Here's how the part is built. I have some questions about the finished solid (model axes, mm). Round coordinates to 2 decimals unless told otherwise and drop trailing zeros. Order: outer loops, then holes, each group sorted by start corner. A loop starts at its lowest first (then second) coordinate and runs counter-clockwise, first axis right, second up. Notation, with made-up numbers: M 48.5,4 L 78.5,4 A16 cw 78.5,8 Z; hole C -13.5,-5.75 d7. An arc over 180 degrees is marked long. Write item = value, one per line. Start each with the question number.
Item 1: I want a section at A-A, the plane z = 0. List the corners of the cut face in (x, y) for me (3 decimals), plus the area to 3 significant figures.
Item 2: Please list where these lines run through material, in increasing order: L1, parallel to Z at x = -0.25, y = -2.8; L2, parallel to X at y = -4.5, z = -0.75; L3, parallel to X at y = -4.1, z = -1.25.
Item 3: I'm going to push flat-ended pins straight in: P1, Ø3, axis at y = -1, z = -1, coming from the -X side; P2, Ø1.5, axis at x = 1.5, y = -3.5, coming from the -Z side; P3, Ø1, axis at x = 3, z = 5.5, coming from the +Y side. Where does each tip first touch, or does it pass through?
Item 4: I want a section at B-B, the plane x = 0. List the corners of the cut face in (y, z) for me (3 decimals), plus the area to 3 significant figures.
Item 5: I want a section at D-D, the plane y = -4.55. List the corners of the cut face in (x, z) for me, plus the area to 3 significant figures.
Item 6: I want a section at C-C, the plane y = -0.25. List the corners of the cut face in (x, z) for me.
Item 7: We'd pull the mould along Z, two halves only. Please class faces 1 (the face through (2, -5, 3)), 2 (the face through (-1.13, -2.49, -0.87)): pulls with the +Z half, pulls with the -Z half, needs draft (parallel to the pull), parting line crosses it, or undercut.
```python
from build123d import *

# Parameters (mm, degrees)
F0_R     = 7.5
F0_R_2   = 1.425
F1_DEPTH = 5
F2_R     = 3
F4_R     = 2


# Not quite as in the source:
# - a fillet or chamfer that OpenCascade refuses, or shapes differently, is made with other operations: its cross-section is extruded or revolved along the edge and cut away or added


with BuildPart() as f1:
    # F0 (on Front) → F1 (new body)
    with BuildSketch(Plane.XZ):
        Circle(F0_R)
        Circle(F0_R_2, mode=Mode.SUBTRACT)
    extrude(amount=F1_DEPTH)

    # F2
    f2_edges = [f1.edges().sort_by_distance(p)[0] for p in [
        (-7.5, 0, 0),
    ]]
    fillet(f2_edges, radius=F2_R)

    # F3: fillet of radius 3 on 1 edges, made by hand

    # F3_s1 → F3_t2 (revolve, cut)
    with BuildSketch(Plane.XY):
        with BuildLine():
            ThreePointArc((7.5, -3), (6.4036236828, -4.4494897428), (4.6715728753, -5))
            Line((4.6715728753, -5), (7.5, -5))
            Line((7.5, -5), (7.5, -3))
        make_face()
    revolve(axis=Axis((0, -5, 0), (0, -1, 0)), mode=Mode.SUBTRACT)

    # F4
    f4_edges = [f1.edges().sort_by_distance(p)[0] for p in [
        (1.425, -2.5, 0),
        (-1.425, 0, 0),
        (-1.425, -5, 0),
    ]]
    fillet(f4_edges, radius=F4_R)


solid = f1.part
```
Filled in:
q1.outline = M -7.5,-3 A3 ccw -4.672,-5 L -3.425,-5 A2 ccw -1.425,-3 L -1.425,-2 A2 ccw -3.425,0 L -4.5,0 A3 ccw Z; M 1.425,-3 A2 ccw 3.425,-5 L 4.672,-5 A3 ccw 7.5,-3 A3 ccw 4.5,0 L 3.425,0 A2 ccw 1.425,-2 Z
q1.area = 50.4 mm^2
q2.L1 = -7.49 to -1.4, 1.4 to 7.49
q2.L2 = -6.29 to -1.96, 1.96 to 6.29
q2.L3 = -6.7 to -1.23, 1.23 to 6.7
q3.P1 = -7.43
q3.P2 = -7.44
q3.P3 = -0.28
q4.outline = M -5,-4.672 A3 ccw -3,-7.5 A3 ccw 0,-4.5 L 0,-3.425 A2 ccw -2,-1.425 L -3,-1.425 A2 ccw -5,-3.425 Z; M -5,3.425 A2 ccw -3,1.425 L -2,1.425 A2 ccw 0,3.425 L 0,4.5 A3 ccw -3,7.5 A3 ccw -5,4.672 Z
q4.area = 50.4 mm^2
q5.outline = C 0,0 d12.5; hole C 0,0 d4.32
q5.area = 108 mm^2
q6.outline = C 0,0 d11.4; hole C 0,0 d4.91
q7.face_1 = needs draft
q7.face_2 = undercut
